Check sheet for the modelled part. Datum: model origin and axes. Units: mm. A direction names the side the tool comes from. Round coordinates to 2 decimals unless told otherwise and drop trailing zeros. Loops run counter-clockwise (first coordinate to the right, second up) from the corner with the lowest first, then second, coordinate; pieces in that order, holes last. Notation, with made-up numbers: (77, 79.25) - (102, 79.25) arc R22 cw to (102, 86.25) - close; hole circle Ø4 at (80.5, 15). An arc over 180 degrees is marked (long way). Put each result on its own line as item: value. Start each with the question number.
```python
from build123d import *

# Parameters (mm, degrees)
BOSS_EXTRUDE1_DEPTH   = 10
BOSS_EXTRUDE1_2_DEPTH = 10
BOSS_EXTRUDE1_3_DEPTH = 10
BOSS_EXTRUDE1_4_DEPTH = 10
BOSS_EXTRUDE2_DEPTH   = 5
FILLET1_R             = 1


with BuildPart() as part:
    # Sketch3 → Boss-Extrude1 (new body)
    with BuildSketch(Plane(origin=(0, 0, 0), x_dir=(1, 0, 0), z_dir=(0, 1, 0))):
        Polygon((-10, -5), (-10, 5), (-12.5, 2.5), (-12.5, -2.5), align=None)
    extrude(amount=BOSS_EXTRUDE1_DEPTH)



with BuildPart() as body_2:
    # Sketch3 → Boss-Extrude1 2 (new body)
    with BuildSketch(Plane(origin=(0, 0, 0), x_dir=(1, 0, 0), z_dir=(0, 1, 0))):
        Polygon((-5, 10), (5, 10), (2.5, 12.5), (-2.5, 12.5), align=None)
    extrude(amount=BOSS_EXTRUDE1_2_DEPTH)


with BuildPart() as body_3:
    # Sketch3 → Boss-Extrude1 3 (new body)
    with BuildSketch(Plane(origin=(0, 0, 0), x_dir=(1, 0, 0), z_dir=(0, 1, 0))):
        Polygon((10, 5), (10, -5), (12.5, -2.5), (12.5, 2.5), align=None)
    extrude(amount=BOSS_EXTRUDE1_3_DEPTH)


with BuildPart() as body_4:
    # Sketch3 → Boss-Extrude1 4 (new body)
    with BuildSketch(Plane(origin=(0, 0, 0), x_dir=(1, 0, 0), z_dir=(0, 1, 0))):
        Polygon((5, -10), (2.5, -12.5), (-2.5, -12.5), (-5, -10), align=None)
    extrude(amount=BOSS_EXTRUDE1_4_DEPTH)


with BuildPart() as part_1:
    add(part.part)

    add(body_2.part)  # Boss-Extrude2 merges body 2

    add(body_3.part)  # Boss-Extrude2 merges body 3

    add(body_4.part)  # Boss-Extrude2 merges body 4
    # Sketch3_4 → Boss-Extrude2 (add)
    # profile 1 of 6: a face of its own
    with BuildSketch(Plane(origin=(0, 0, 0), x_dir=(1, 0, 0), z_dir=(0, 1, 0))):
        with BuildLine():
            Line((-9.5, 12.5), (-2.5, 12.5))
            Line((-2.5, 12.5), (-5, 10))
            Line((-5, 10), (5, 10))
            Line((5, 10), (2.5, 12.5))
            Line((2.5, 12.5), (9.5, 12.5))
            ThreePointArc((9.5, 12.5), (11.621320344, 11.621320344), (12.5, 9.5))
            Line((12.5, 9.5), (12.5, 2.5))
            Line((12.5, 2.5), (10, 5))
            Line((10, 5), (10, -5))
            Line((10, -5), (12.5, -2.5))
            Line((12.5, -2.5), (12.5, -9.5))
            ThreePointArc((12.5, -9.5), (11.621320344, -11.621320344), (9.5, -12.5))
            Line((9.5, -12.5), (2.5, -12.5))
            Line((2.5, -12.5), (5, -10))
            Line((5, -10), (-5, -10))
            Line((-5, -10), (-2.5, -12.5))
            Line((-2.5, -12.5), (-9.5, -12.5))
            ThreePointArc((-9.5, -12.5), (-11.621320344, -11.621320344), (-12.5, -9.5))
            Line((-12.5, -9.5), (-12.5, -2.5))
            Line((-12.5, -2.5), (-10, -5))
            Line((-10, -5), (-10, 5))
            Line((-10, 5), (-12.5, 2.5))
            Line((-12.5, 2.5), (-12.5, 9.5))
            ThreePointArc((-12.5, 9.5), (-11.621320344, 11.621320344), (-9.5, 12.5))
        make_face()
        Polygon((-5, -7.5), (-7.5, -5), (-7.5, 5), (-5, 7.5), (5, 7.5), (7.5, 5), (7.5, -5), (5, -7.5), align=None, mode=Mode.SUBTRACT)
    # profile 2 of 6: a face of its own
    with BuildSketch(Plane(origin=(0, 0, 0), x_dir=(1, 0, 0), z_dir=(0, 1, 0))):
        Polygon((-7.5, -5), (-7.5, 5), (-5, 7.5), (5, 7.5), (7.5, 5), (7.5, -5), (5, -7.5), (-5, -7.5), align=None)
    # profile 3 of 6: a face of its own
    with BuildSketch(Plane(origin=(0, 0, 0), x_dir=(1, 0, 0), z_dir=(0, 1, 0))):
        Polygon((5, -10), (2.5, -12.5), (-2.5, -12.5), (-5, -10), align=None)
    # profile 4 of 6: a face of its own
    with BuildSketch(Plane(origin=(0, 0, 0), x_dir=(1, 0, 0), z_dir=(0, 1, 0))):
        Polygon((-10, -5), (-10, 5), (-12.5, 2.5), (-12.5, -2.5), align=None)
    # profile 5 of 6: a face of its own
    with BuildSketch(Plane(origin=(0, 0, 0), x_dir=(1, 0, 0), z_dir=(0, 1, 0))):
        Polygon((-5, 10), (5, 10), (2.5, 12.5), (-2.5, 12.5), align=None)
    # profile 6 of 6: a face of its own
    with BuildSketch(Plane(origin=(0, 0, 0), x_dir=(1, 0, 0), z_dir=(0, 1, 0))):
        Polygon((10, 5), (10, -5), (12.5, -2.5), (12.5, 2.5), align=None)
    extrude(amount=-BOSS_EXTRUDE2_DEPTH)

    # Fillet1
    fillet1_edges = [part_1.edges().sort_by_distance(p)[0] for p in [
        (-11.621320344, -5, -11.621320344),
        (-12.5, -5, 0),
        (0, -5, -12.5),
        (11.621320344, -5, -11.621320344),
        (12.5, -5, 0),
        (11.621320344, -5, 11.621320344),
        (0, -5, 12.5),
        (-11.621320344, -5, 11.621320344),
    ]]
    fillet(fillet1_edges, radius=FILLET1_R)


solid = part_1.part
```
Q1. Cross-section at C-C on z = -1.75. Enter the section's corners in (x, y).
Q2. Cross-section at A-A on y = 5.5. Enter the section's corners in (x, z).
Q3. Draft check along Z on faces 5 (the face through (-4, 5, -11)), 6 (the face through (-12.199, -4.715, -0.133)), 7 (the face through (0, 5, 10)), 8 (the face through (0, 0, 0)). Enter one of: +Z half, -Z half, draft (parallel to the pull), parting line (faces both ways), or undercut.
Q4. Set-up check for faces 1 (the face through (-11, 5, -4)), 2 (the face through (-4, 5, 11)), 3 (the face through (0, 5, -10)), 4 (the face through (10, 5, 0)): record each of +Z, -Z, +X, -X, +Y, -Y from which the full face is reachable in a straight line by a thin tool's end or side.
Q5. Cross-section at B-B on x = -4. Enter the section's corners in (y, z), and give its area (3 significant figures).
Q6. Material ranges on line 1 (Z direction, x = -0.5, y = 4.25); line 2 (Z direction, x = 3.5, y = 1.5), recorded low to high. Write a range as from..to.
Q7. Depth check by flat-ended pin: pin 1 Ø8 at (y, z) = (7.5, -10) entering from +X. Enter the tip coordinate at first touch or a pass-through.
Q8. Cross-section at D-D on x = 0.25. Enter the section's corners in (y, z).
Answer list:
1. outline: (-12.5, -4) arc R1 ccw to (-11.5, -5) - (11.5, -5) arc R1 ccw to (12.5, -4) - (12.5, 10) - (10, 10) - (10, 0) - (-10, 0) - (-10, 10) - (-12.5, 10) - close
2. outline: (-12.5, -2.5) - (-10, -5) - (-10, 5) - (-12.5, 2.5) - close; (-5, -10) - (-2.5, -12.5) - (2.5, -12.5) - (5, -10) - close; (-5, 10) - (5, 10) - (2.5, 12.5) - (-2.5, 12.5) - close; (10, -5) - (12.5, -2.5) - (12.5, 2.5) - (10, 5) - close
3. face 5: -Z half
3. face 6: draft
3. face 7: undercut
3. face 8: undercut
4. face 1: -Z, -X, +Y
4. face 2: +Z, -X, +Y
4. face 3: +X, -X, +Y
4. face 4: +Z, -Z, +Y
5. outline: (-5, -11.5) arc R1 ccw to (-4, -12.5) - (0, -12.5) - (0, -11) - (10, -11) - (10, -10) - (0, -10) - (0, 10) - (10, 10) - (10, 11) - (0, 11) - (0, 12.5) - (-4, 12.5) arc R1 ccw to (-5, 11.5) - close
5. area: 145 mm2
6. line 1: z = -12.5..-10, 10..12.5
6. line 2: z = -11.5..-10, 10..11.5
7. pin 1: stops at x = 5
8. outline: (-5, -11.5) arc R1 ccw to (-4, -12.5) - (10, -12.5) - (10, -10) - (0, -10) - (0, 10) - (10, 10) - (10, 12.5) - (-4, 12.5) arc R1 ccw to (-5, 11.5) - close
